Design review of the part built by this model. Coordinates are the model's own, in mm. Face numbers are marked on the shaded views. A direction names the side the tool comes from. Give positions to 0.01 mm unless a question says otherwise; leave off trailing zeros. Write each loop counter-clockwise with the first axis right and the second up, starting at its lowest first coordinate (ties: lowest second). Pieces come first, ordered by that corner, then holes.
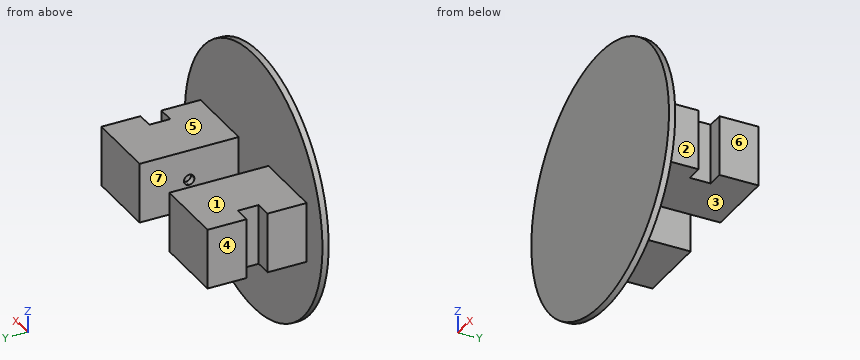
```python
from build123d import *

# Parameters (mm, degrees)
SKETCH_1_W               = 34.7
SKETCH_1_H               = 47.5
EXTRUDE_1_DEPTH          = 29
EXTRUDE_1_2_DEPTH        = 29
SKETCH_2_W               = 29
SKETCH_2_H               = 10
CUT_EXTRUDE_1_DEPTH      = 8
SKETCH_3_W               = 29
SKETCH_3_H               = 10
CUT_EXTRUDE_2_DEPTH      = 8
SKETCH_4_R               = 62.5
EXTRUDE_2_DEPTH          = 3
CUT_EXTRUDE_3_DEPTH      = 22
CUT_EXTRUDE_3_DEPTH_BACK = 3
SKETCH_5_R               = 2.5
CUT_EXTRUDE_START        = -3
CUT_EXTRUDE_4_DEPTH      = 3


with BuildPart() as part:
    # Sketch 1 → Extrude 1 (new body)
    with BuildSketch(Plane.XY):
        with Locations((17.35, 23.75)):
            Rectangle(SKETCH_1_W, SKETCH_1_H)
    extrude(amount=EXTRUDE_1_DEPTH)

    # Sketch 2 → Cut-Extrude 1 (cut)
    with BuildSketch(Plane(origin=(34.7, 0, 0), x_dir=(0, 0, -1), z_dir=(1, 0, 0))):
        with Locations((-14.5, 23.75)):
            Rectangle(SKETCH_2_W, SKETCH_2_H)
    extrude(amount=-CUT_EXTRUDE_1_DEPTH, mode=Mode.SUBTRACT)



with BuildPart() as body_2:
    # Sketch 1 → Extrude 1 2 (new body)
    with BuildSketch(Plane.XY):
        with Locations((-44.35, 23.75)):
            Rectangle(SKETCH_1_W, SKETCH_1_H)
    extrude(amount=EXTRUDE_1_2_DEPTH)

    # Sketch 3 → Cut-Extrude 2 (cut)
    with BuildSketch(Plane.ZY.offset(61.7)):
        with Locations((14.5, 23.75)):
            Rectangle(SKETCH_3_W, SKETCH_3_H)
    extrude(amount=-CUT_EXTRUDE_2_DEPTH, mode=Mode.SUBTRACT)


with BuildPart() as part_1:
    add(part.part)

    add(body_2.part)  # Extrude 2 merges body 2
    # Sketch 4 → Extrude 2 (add)
    with BuildSketch(Plane.XZ):
        with Locations(Location((-13.5, 14.5, 0), (0, 0, 270))):
            Circle(SKETCH_4_R)
    extrude(amount=EXTRUDE_2_DEPTH)

    # Sketch 5 → Cut-Extrude 3 (cut, two sides: drawn at the far end of the back side and taken through both)
    with BuildSketch(Plane(origin=(-27, 0, 0), x_dir=(0, 0, -1), z_dir=(1, 0, 0)).offset(-CUT_EXTRUDE_3_DEPTH_BACK)):
        with Locations(Location((-14.5, 23.75, 0), (0, 0, 180))):
            Circle(SKETCH_5_R)
    extrude(amount=CUT_EXTRUDE_3_DEPTH + CUT_EXTRUDE_3_DEPTH_BACK, mode=Mode.SUBTRACT)

    # Sketch 6 → Cut-Extrude 4 (cut)
    with BuildSketch(Plane.ZY.offset(CUT_EXTRUDE_START)):
        with BuildLine():
            ThreePointArc((17, 23.75), (16.267766953, 25.517766953), (14.5, 26.25))
            Line((14.5, 26.25), (14.5, 23.75))
            Line((14.5, 23.75), (17, 23.75))
        make_face()
        with BuildLine():
            Line((14.5, 23.75), (14.5, 26.25))
            ThreePointArc((14.5, 26.25), (12.732233047, 25.517766953), (12, 23.75))
            Line((12, 23.75), (14.5, 23.75))
        make_face()
        with BuildLine():
            Line((17, 23.75), (14.5, 23.75))
            Line((14.5, 23.75), (14.5, 21.25))
            ThreePointArc((14.5, 21.25), (16.267766953, 21.982233047), (17, 23.75))
        make_face()
        with BuildLine():
            Line((14.5, 21.25), (14.5, 23.75))
            Line((14.5, 23.75), (12, 23.75))
            ThreePointArc((12, 23.75), (12.732233047, 21.982233047), (14.5, 21.25))
        make_face()
    extrude(amount=CUT_EXTRUDE_4_DEPTH, mode=Mode.SUBTRACT)


solid = part_1.part
```
(1) Mouldability with a two-part tool opening along X and no side actions: class the marked faces 5, 6 and 7 as pulls with the +X half, pulls with the -X half, needs draft (parallel to the pull), parting line crosses it, or undercut.
Resolved:
face 5: needs draft
face 6: pulls with the +X half
face 7: undercut
(2) To check wall thickness, follow L1, parallel to X at y = 43, z = 23; L2, parallel to Y at x = -28.1, z = 14.5; L3, parallel to X at y = 25, z = 4. State the ranges of each line that lie inside material, in increasing order.
Resolved:
L1: x = -61.7 to -27, 0 to 34.7
L2: y = -3 to 21.25, 26.25 to 47.5
L3: x = -53.7 to -27, 0 to 26.7
(3) Tool access review of the marked faces 1, 2, 3 and 4: name each direction out of +Z, -Z, +X, -X, +Y, -Y from which nothing blocks a thin tool from reaching the whole face with its end or side.
Resolved:
face 1: +Z, +X, -X, +Y
face 2: +Z, -Z, +X, +Y
face 3: -Z, +X, -X, +Y
face 4: +Z, -Z, -X, +Y
(4) Clearance check with flat-ended pins moving along their axes: P1, Ø17.5, axis at x = -38, y = 33.5, coming from the -Z side; P2, Ø6, axis at y = 9.5, z = 22.5, coming from the -X side; P3, Ø1.5, axis at y = 25, z = 14, coming from the -X side. State where each tip first meets the part, or that it passes through.
Resolved:
P1: stops at z = 0
P2: stops at x = -61.7
P3: stops at x = -53.7
(5) Consider section D-D, the plane x = -13.5. Give the boundary of the cut face in (y, z), then the cut area to 3 significant figures.
Resolved:
outline: (-3, -48) - (0, -48) - (0, 77) - (-3, 77) - close
area: 375 mm2
(6) Consider section A-A, the plane x = 33. Give the boundary of the cut face in (y, z).
Resolved:
outline: (-3, -27.26) - (0, -27.26) - (0, 0) - (18.75, 0) - (18.75, 29) - (0, 29) - (0, 56.26) - (-3, 56.26) - close; (28.75, 0) - (47.5, 0) - (47.5, 29) - (28.75, 29) - close
(7) Consider section C-C, the plane x = 6.5. Give the boundary of the cut face in (y, z).
Resolved:
outline: (-3, -44.71) - (0, -44.71) - (0, 0) - (47.5, 0) - (47.5, 29) - (0, 29) - (0, 73.71) - (-3, 73.71) - close
(8) Consider section B-B, the plane z = 3.5. Give the boundary of the cut face in (x, y).
Resolved:
outline: (-75.02, -3) - (48.02, -3) - (48.02, 0) - (34.7, 0) - (34.7, 18.75) - (26.7, 18.75) - (26.7, 28.75) - (34.7, 28.75) - (34.7, 47.5) - (0, 47.5) - (0, 0) - (-27, 0) - (-27, 47.5) - (-61.7, 47.5) - (-61.7, 28.75) - (-53.7, 28.75) - (-53.7, 18.75) - (-61.7, 18.75) - (-61.7, 0) - (-75.02, 0) - close
